from build123d import *

# Parameters (mm, degrees)
SKETCH4_R               = 17.5
SKETCH4_R_2             = 2
BOSS_EXTRUDE1_DEPTH     = 2
SKETCH5_R               = 8
BOSS_EXTRUDE2_DEPTH     = 5
SKETCH6_R               = 2.1
CUT_EXTRUDE1_DEPTH      = 6
CUT_EXTRUDE1_DEPTH_BACK = 1


with BuildPart() as part:
    # Sketch4 → Boss-Extrude1 (new body)
    with BuildSketch(Plane(origin=(0, 0, 0), x_dir=(1, 0, 0), z_dir=(0, 1, 0))):
        Circle(SKETCH4_R)
        with Locations((10.87, 0)):
            Circle(SKETCH4_R_2, mode=Mode.SUBTRACT)
        with Locations((0, -10.87)):
            Circle(SKETCH4_R_2, mode=Mode.SUBTRACT)
        with Locations((-10.87, 0)):
            Circle(SKETCH4_R_2, mode=Mode.SUBTRACT)
        with Locations((0, 10.87)):
            Circle(SKETCH4_R_2, mode=Mode.SUBTRACT)
    extrude(amount=BOSS_EXTRUDE1_DEPTH)

    # Sketch5 → Boss-Extrude2 (add)
    with BuildSketch(Plane(origin=(0, 0, 0), x_dir=(-1, 0, 0), z_dir=(0, 1, 0))):
        Circle(SKETCH5_R)
        Polygon((-6.1, -3.521836642), (0, -7.043673284), (6.1, -3.521836642), (6.1, 3.521836642), (0, 7.043673284), (-6.1, 3.521836642), align=None, mode=Mode.SUBTRACT)
    extrude(amount=BOSS_EXTRUDE2_DEPTH)

    # Sketch6 → Cut-Extrude1 (cut, two sides)
    with BuildSketch(Plane(origin=(0, 0, 0), x_dir=(1, 0, 0), z_dir=(0, 1, 0))) as cut_extrude1_sk:
        Circle(SKETCH6_R)
    extrude(amount=CUT_EXTRUDE1_DEPTH, mode=Mode.SUBTRACT)
    extrude(cut_extrude1_sk.sketch, amount=-CUT_EXTRUDE1_DEPTH_BACK, mode=Mode.SUBTRACT)


solid = part.part
Geometry check sheet. Reference: the model listing, model coordinates, mm. A direction names the side the tool comes from. Give positions to 0.01 mm unless a question says otherwise; leave off trailing zeros. Loops run counter-clockwise (first coordinate to the right, second up) from the corner with the lowest first, then second, coordinate; pieces in that order, holes last. Notation, with made-up numbers: (66.25, 2) -> (109.25, 2) arc R25 cw to (109.25, 28) -> close; hole circle Ø8 at (85, 47.5). An arc over 180 degrees is marked (long way). Answer in a Markdown table with one row per item. Add a question column.
1) Cross-section at D-D on z = 10.87. Record the boundary of the cut face in (x, y).
2) Cross-section at A-A on z = 1. Record the boundary of the cut face in (x, y).
3) Set-up check for faces 1 (the face through (-0.26, 0.986, 8.887)), 2 (the face through (-3, 2, 0)): record each of +Z, -Z, +X, -X, +Y, -Y from which the full face is reachable in a straight line by a thin tool's end or side.
4) Draft check along X on faces 3 (the face through (3.007, 3.479, 5.307)), 4 (the face through (4, 2, 8)), 5 (the face through (6.1, 3, 0)), 6 (the face through (1.73, 3.48, -7.81)). Enter one of: pulls with the +X half, pulls with the -X half, needs draft (parallel to the pull), parting line crosses it, or undercut.
5) Material ranges on probe 1 along Z at (x, y) = (0, 0.5); probe 2 along Z at (x, y) = (0, 2.5), recorded low to high. Write a range as from..to.
6) Cross-section at C-C on x = 11. Record the boundary of the cut face in (y, z).
7) Cross-section at B-B on y = 4.4. Record the boundary of the cut face in (x, z).
8) Gauge pin test, flat ends, axial feed: P1, Ø12, axis at x = 14, z = -6, coming from the +Y side; P2, Ø2.5, axis at x = 0, z = 0, coming from the -Y side; P3, Ø3, axis at x = -2, y = 0.5, coming from the +Z side; P4, Ø1.5, axis at y = 4, z = -1, coming from the -X side. Record the tip position at first contact, or that the pin passes through.
Outcome:
| question | item | result |
|---|---|---|
| 1 | outline | (-13.71, 0) -> (-2, 0) -> (-2, 2) -> (-13.71, 2) -> close; (2, 0) -> (13.71, 0) -> (13.71, 2) -> (2, 2) -> close |
| 2 | outline | (-17.47, 0) -> (-12.6, 0) -> (-12.6, 2) -> (-17.47, 2) -> close; (-9.14, 0) -> (-1.85, 0) -> (-1.85, 2) -> (-6.1, 2) -> (-6.1, 5) -> (-7.94, 5) -> (-7.94, 2) -> (-9.14, 2) -> close; (1.85, 0) -> (9.14, 0) -> (9.14, 2) -> (7.94, 2) -> (7.94, 5) -> (6.1, 5) -> (6.1, 2) -> (1.85, 2) -> close; (12.6, 0) -> (17.47, 0) -> (17.47, 2) -> (12.6, 2) -> close |
| 3 | face 1 | +Y, -Y |
| 3 | face 2 | +Y |
| 4 | face 3 | undercut |
| 4 | face 4 | needs draft |
| 4 | face 5 | undercut |
| 4 | face 6 | parting line crosses it |
| 5 | probe 1 | z = -17.5..-12.87, -8.87..-2.1, 2.1..8.87, 12.87..17.5 |
| 5 | probe 2 | z = -8..-7.04, 7.04..8 |
| 6 | outline | (0, -13.61) -> (2, -13.61) -> (2, -2) -> (0, -2) -> close; (0, 2) -> (2, 2) -> (2, 13.61) -> (0, 13.61) -> close |
| 7 | outline | circle Ø16 at (0, 0); hole (-6.1, -3.52) -> (0, -7.04) -> (6.1, -3.52) -> (6.1, 3.52) -> (0, 7.04) -> (-6.1, 3.52) -> close |
| 8 | P1 | stops at y = 2 |
| 8 | P2 | passes through |
| 8 | P3 | stops at z = 17.49 |
| 8 | P4 | stops at x = -8 |
